Input: part model. Units: mm. Frame: model coordinates. Coordinates: 2 decimals unless noted, no trailing zeros. Loops run counter-clockwise (first coordinate to the right, second up) from the corner with the lowest first, then second, coordinate; pieces in that order, holes last. Notation, with made-up numbers: M 60.5,1.5 L 68.5,1.5 A14 cw 68.5,5.5 Z; hole C -18.75,83 d5. An arc over 180 degrees is marked long. Use a Markdown table: item, result. Add a question column.
1. Section A-A on x = 0. Output: boundary loops of the cut face in (y, z).
2. Line query: L1, parallel to Y at x = 0.75, z = 208; L2, parallel to X at y = -1, z = 222; L3, parallel to Y at x = 0, z = 123. Output: solid intervals per line, ascending. Write a range as [from, to].
3. Draft query along X for faces 1 (the flat face through (2, 5, 0)), 2 (the cylindrical face through (5.718, 1.801, 225.4)), 3 (the cylindrical face through (-0.64, 4.91, 225.76)). Return one class per face: +X half, -X half, draft (parallel to the pull), parting line (faces both ways), or undercut.
4. Pin query (flat end, axial travel): pin 1 (3 mm diameter, centred on y = 2.5, z = 88.5, fed in from -X); pin 2 (3 mm diameter, centred on y = 0, z = 452.44, fed in from -X); pin 3 (5 mm diameter, centred on y = 4, z = 399, fed in from +X). Return the tip coordinate at first contact, or that it passes through.
5. Section B-B on z = 391. Output: boundary loops of the cut face in (x, y), then the cut area to 3 significant figures.
```python
from build123d import *

# Parameters (mm, degrees)
SKETCH1_R                    = 5.9944
SKETCH1_R_2                  = 4.953
BOSS_EXTRUDE1_DEPTH          = 457.2
SKETCH8_R                    = 5.1435
CUT_EXTRUDE2_DEPTH           = 25.4
CUT_EXTRUDE3_START           = -25.4
SKETCH9_R                    = 5.1435
CUT_EXTRUDE3_DEPTH           = 25.4
F_1_8_0_125_DIAMETER_HOLE1_D = 3.175


with BuildPart() as part:
    # Sketch1 → Boss-Extrude1 (new body)
    with BuildSketch(Plane.XY):
        Circle(SKETCH1_R)
        Circle(SKETCH1_R_2, mode=Mode.SUBTRACT)
    extrude(amount=BOSS_EXTRUDE1_DEPTH)

    # Sketch8 → Cut-Extrude2 (cut)
    with BuildSketch(Plane(origin=(0, 0, 0), x_dir=(-1, 0, 0), z_dir=(0, 0, -1))):
        Circle(SKETCH8_R)
    extrude(amount=-CUT_EXTRUDE2_DEPTH, mode=Mode.SUBTRACT)

    # Sketch9 → Cut-Extrude3 (cut)
    with BuildSketch(Plane.XY.offset(457.2).offset(CUT_EXTRUDE3_START)):
        with Locations(Location((0, 0, 0), (0, 0, 180))):
            Circle(SKETCH9_R)
    extrude(amount=CUT_EXTRUDE3_DEPTH, mode=Mode.SUBTRACT)

    # 1/8 (0.125) Diameter Hole1 (through all)
    with Locations(Plane.ZY.offset(5.9944)):
        with Locations((452.4375, 0), (4.7625, 0)):
            Hole(F_1_8_0_125_DIAMETER_HOLE1_D / 2)


solid = part.part
```
Answers below:
| question | item | result |
|---|---|---|
| 1 | outline | M -5.99,0 L -5.14,0 L -5.14,25.4 L -4.95,25.4 L -4.95,431.8 L -5.14,431.8 L -5.14,457.2 L -5.99,457.2 Z; M 4.95,25.4 L 5.14,25.4 L 5.14,0 L 5.99,0 L 5.99,457.2 L 5.14,457.2 L 5.14,431.8 L 4.95,431.8 Z |
| 2 | L1 | y = [-5.95, -4.9], [4.9, 5.95] |
| 2 | L2 | x = [-5.91, -4.85], [4.85, 5.91] |
| 2 | L3 | y = [-5.99, -4.95], [4.95, 5.99] |
| 3 | face 1 | draft |
| 3 | face 2 | parting line |
| 3 | face 3 | undercut |
| 4 | pin 1 | stops at x = -5.91 |
| 4 | pin 2 | passes through |
| 4 | pin 3 | stops at x = 5.8 |
| 5 | outline | C 0,0 d11.99; hole C 0,0 d9.91 |
| 5 | area | 35.8 mm² |
